```python
from build123d import *

# Parameters (mm, degrees)
F0_R      = 1.7
F1_DEPTH  = 1.65
F2_W      = 9
F2_H      = 1.65
F3_DEPTH  = 11
F5_DEPTH  = 10
F6_W      = 0.6
F6_H      = 6.1
F7_DEPTH  = 8.5
F8_W      = 12.3
F8_H      = 10.15
F8_H_2    = 6.25
F9_DEPTH  = 10.9
F10_W     = 2.35
F10_H     = 25.75
F10_H_2   = 20.7
F10_W_2   = 46.2
F10_H_3   = 5
F10_H_4   = 20.8
F11_DEPTH = 8.5


with BuildPart() as f1:
    # F0 (on Top) → F1 (new body)
    with BuildSketch(Plane.XY):
        Polygon((-26.7, -48.25), (-25.7, -48.25), (14.6, -48.25), (26.7, -48.25), (26.7, 50.85), (-26.7, 50.85), align=None)
        with Locations((-24.4879107922, -46.4384518564)):
            Circle(F0_R, mode=Mode.SUBTRACT)
        with Locations((-18.5, -15.5)):
            Circle(F0_R, mode=Mode.SUBTRACT)
        with Locations((24.6273092926, -39.5274497569)):
            Circle(F0_R, mode=Mode.SUBTRACT)
        with Locations((9.15, -15.5)):
            Circle(F0_R, mode=Mode.SUBTRACT)
        with Locations((-24.4879107922, 36.1)):
            Circle(F0_R, mode=Mode.SUBTRACT)
        with Locations((24.6273092926, 36.1)):
            Circle(F0_R, mode=Mode.SUBTRACT)
        Polygon((-25.7, -48.25), (-23.1, -50.85), (12, -50.85), (14.6, -48.25), align=None)
    extrude(amount=F1_DEPTH)

    # F2 (on face) → F3 (join)
    with BuildSketch(Plane.XY.offset(1.65)):
        with Locations((-18.2, 50.025)):
            Rectangle(F2_W, F2_H)
        with Locations((-18.2, 51.675)):
            Rectangle(F2_W, F2_H)
    extrude(amount=F3_DEPTH)

    # F4 (on face) → F5 (join)
    with BuildSketch(Plane.XZ.offset(-49.2)):
        with BuildLine():
            Line((-14.3, 1.65), (-14.3, 7.75))
            ThreePointArc((-14.3, 7.75), (-18.2, 11.65), (-22.1, 7.75))
            Line((-22.1, 7.75), (-22.1, 1.65))
            Line((-22.1, 1.65), (-14.3, 1.65))
        make_face()
    extrude(amount=F5_DEPTH)

    # F6 (on face) → F7 (join)
    with BuildSketch(Plane.XZ.offset(-49.2)):
        with Locations((-22.4, 4.7)):
            Rectangle(F6_W, F6_H)
        with Locations((-14, 4.7)):
            Rectangle(F6_W, F6_H)
    extrude(amount=F7_DEPTH)

    # F8 (on face) → F9 (join)
    with BuildSketch(Plane.XY.offset(1.65)):
        with Locations((11.95, 45.775)):
            Rectangle(F8_W, F8_H)
        with Locations((11.95, 53.975)):
            Rectangle(F8_W, F8_H_2)
    extrude(amount=F9_DEPTH)

    # F10 (on face) → F11 (join)
    with BuildSketch(Plane.XY.offset(1.65)):
        with Locations((24.525, 20.525)):
            Rectangle(F10_W, F10_H)
        with Locations((24.525, -3.7)):
            Rectangle(F10_W, F10_H_2)
        with Locations((24.525, -26.4774497569)):
            Rectangle(F10_W, F10_H_2)
        with Locations((2.6, -44.75)):
            Rectangle(F10_W_2, F10_H_3)
        with Locations((-24.525, -33.3384518564)):
            Rectangle(F10_W, F10_H_4)
        with Locations((-24.525, -10.5384518564)):
            Rectangle(F10_W, F10_H_4)
        with Locations((-24.525, 12.4115481436)):
            Rectangle(F10_W, F10_H_4)
    extrude(amount=F11_DEPTH)


solid = f1.part
```
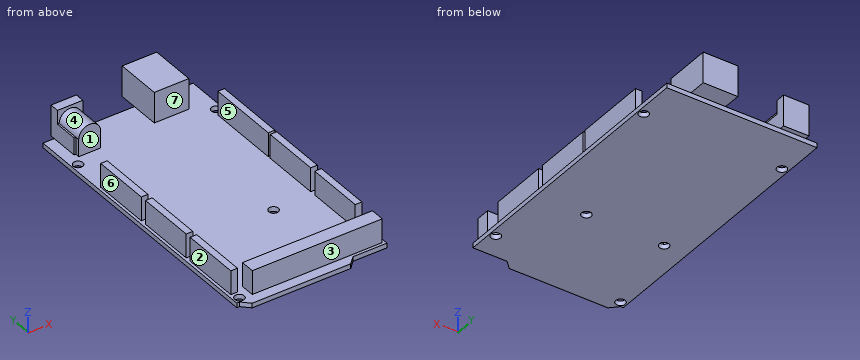
Geometry: final body of the model. Coordinates: model frame, mm. Face numbers are marked on the shaded views. A direction names the side the tool comes from. Give positions to 0.01 mm unless a question says otherwise; leave off trailing zeros. Order: outer loops, then holes, each group sorted by start corner. A loop starts at its lowest first (then second) coordinate and runs counter-clockwise, first axis right, second up. Notation, with made-up numbers: (38.5, 50.25) -> (79.5, 50.25) arc R17 ccw to (79.5, 81.25) -> close; hole circle Ø11 at (-23, -20.75). An arc over 180 degrees is marked (long way). Write each question's results on one line, items separated by ' | '. Start each with the question number.
1) Section B-B (y = 36.1). Return loops of the section in (x, z).
2) Section A-A (x = 9.15). Return loops of the section in (y, z), then the cut area to 3 significant figures.
3) Set-up query: the marked faces 1, 2 and 3. Return all of +Z, -Z, +X, -X, +Y, -Y with unobstructed straight access to the full face (end or side cutting, diameter ignored); none if empty.
4) First-contact query: pin 1 (2.5 mm diameter, centred on x = 6, z = 8, fed in from -Y); pin 2 (2.5 mm diameter, centred on y = -44, z = 8, fed in from +X); pin 3 (4 mm diameter, centred on y = -33.5, z = 4.5, fed in from -X). Flat tips, straight axial feed; report the tip coordinate or a pass-through.
5) Section C-C (y = -24). Return loops of the section in (x, z).
6) Section D-D (z = 5.5). Count the separate pieces of the cut face and the enclosed holes in it, then the cut area to 3 significant figures.
7) Line query: line 1 (Y direction, x = -23.5, z = 5.5); line 2 (X direction, y = -34, z = 8.5); line 3 (Y direction, x = 8.5, z = 5.25). Output: solid intervals per line, ascending. Write a range as from..to.
8) Draft query along X for the marked faces 4, 5, 6 and 7. Return one class per face: pulls with the +X half, pulls with the -X half, needs draft (parallel to the pull), parting line crosses it, or undercut.
Calculated:
1) outline: (-26.7, 0) -> (-26.19, 0) -> (-26.19, 1.65) -> (-26.7, 1.65) -> close; (-22.79, 0) -> (22.93, 0) -> (22.93, 1.65) -> (-22.79, 1.65) -> close; (26.33, 0) -> (26.7, 0) -> (26.7, 1.65) -> (26.33, 1.65) -> close
2) outline: (-50.85, 0) -> (-17.2, 0) -> (-17.2, 1.65) -> (-42.25, 1.65) -> (-42.25, 10.15) -> (-47.25, 10.15) -> (-47.25, 1.65) -> (-50.85, 1.65) -> close; (-13.8, 0) -> (50.85, 0) -> (50.85, 1.65) -> (57.1, 1.65) -> (57.1, 12.55) -> (40.7, 12.55) -> (40.7, 1.65) -> (-13.8, 1.65) -> close | area: 383 mm2
3) face 1: +Z, +X, -X | face 2: +Z, -X, +Y, -Y | face 3: +Z, +X, -X, -Y
4) pin 1: y = -47.25 | pin 2: x = 25.7 | pin 3: x = -25.7
5) outline: (-26.7, 0) -> (26.7, 0) -> (26.7, 1.65) -> (25.7, 1.65) -> (25.7, 10.15) -> (23.35, 10.15) -> (23.35, 1.65) -> (-23.35, 1.65) -> (-23.35, 10.15) -> (-25.7, 10.15) -> (-25.7, 1.65) -> (-26.7, 1.65) -> close
6) separate pieces: 9 | enclosed holes: 0 | area: 855 mm2
7) line 1: -43.74..-22.94, -20.94..-0.14, 2.01..22.81 | line 2: -25.7..-23.35, 23.35..25.7 | line 3: -47.25..-42.25, 40.7..57.1
8) face 4: undercut | face 5: undercut | face 6: pulls with the -X half | face 7: needs draft
